Input: dimensioned drawing with shaded views. Units: mm. Origin: part minimum x, y, z. A direction names the side the tool comes from. Coordinates: 2 decimals unless noted, no trailing zeros. Loops run counter-clockwise (first coordinate to the right, second up) from the corner with the lowest first, then second, coordinate; pieces in that order, holes last. Notation, with made-up numbers: (31.25, 48) - (51.25, 48) arc R16 ccw to (51.25, 71) - close; hole circle Ø2 at (14.5, 79). An arc over 180 degrees is marked (long way). Put each result on its own line as item: value. Start each with the question number.
1) Section B-B on x = 8. Output: boundary loops of the cut face in (y, z), and give its area (3 significant figures).
2) Section D-D on z = 4.75. Output: boundary loops of the cut face in (x, y).
3) Section C-C on y = 2. Output: boundary loops of the cut face in (x, z).
4) Section A-A on z = 8. Output: boundary loops of the cut face in (x, y).
5) Contact query for flat-ended pins moving along their axis: pin 1 Ø1.5 at (y, z) = (5.5, 11.5) entering from +X; pin 2 Ø1.5 at (x, z) = (9, 18) entering from +Y; pin 3 Ø3.5 at (x, z) = (8, 6) entering from +Y. Output: stop coordinate, or through.
6) Material intervals for line 1 along Z through (x, y) = (8, 4.75); line 2 along Z through (x, y) = (8, 1.25); line 3 along Y through (x, z) = (8, 23), sorted ascending. Write a range as from..to.
7) Reachability of the marked faces 5, 6 and 7 from +Z, -Z, +X, -X, +Y, -Y: full face, straight path, thin tool, end or side. Return the list, or none.
8) Draft query along Z for the marked faces 1, 2, 3 and 4. Return one class per face: +Z half, -Z half, draft (parallel to the pull), parting line (faces both ways), or undercut.
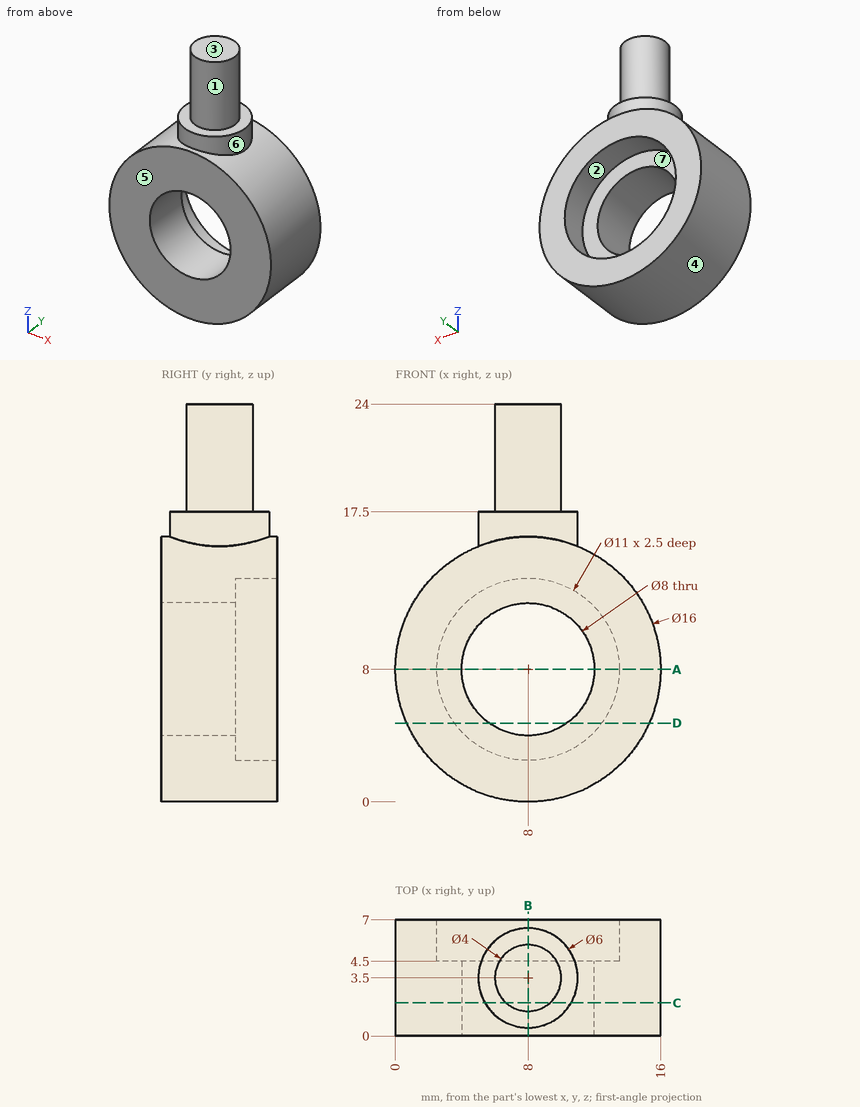
Answer block:
1. outline: (0, 0) - (7, 0) - (7, 2.5) - (4.5, 2.5) - (4.5, 4) - (0, 4) - close; (0, 12) - (4.5, 12) - (4.5, 13.5) - (7, 13.5) - (7, 16) - (6.5, 16) - (6.5, 17.5) - (5.5, 17.5) - (5.5, 24) - (1.5, 24) - (1.5, 17.5) - (0.5, 17.5) - (0.5, 16) - (0, 16) - close
1. area: 83.5 mm²
2. outline: (0.69, 0) - (5.67, 0) - (5.67, 4.5) - (3.56, 4.5) - (3.56, 7) - (0.69, 7) - close; (10.33, 0) - (15.31, 0) - (15.31, 7) - (12.44, 7) - (12.44, 4.5) - (10.33, 4.5) - close
3. outline: (5.4, 15.57) arc R8 ccw (long way) to (10.6, 15.57) - (10.6, 17.5) - (9.32, 17.5) - (9.32, 24) - (6.68, 24) - (6.68, 17.5) - (5.4, 17.5) - close; hole circle Ø8 at (8, 8)
4. outline: (0, 0) - (4, 0) - (4, 4.5) - (2.5, 4.5) - (2.5, 7) - (0, 7) - close; (12, 0) - (16, 0) - (16, 7) - (13.5, 7) - (13.5, 4.5) - (12, 4.5) - close
5. pin 1: stops at x = 15.51
5. pin 2: stops at y = 6.47
5. pin 3: passes through
6. line 1: z = 0..2.5, 13.5..24
6. line 2: z = 0..4, 12..17.5
6. line 3: y = 1.5..5.5
7. face 5: +Z, -Z, +X, -X, -Y
7. face 6: +Z
7. face 7: +Y
8. face 1: draft
8. face 2: undercut
8. face 3: +Z half
8. face 4: parting line
